from build123d import *


# Not quite as in the source:
# - a fillet or chamfer that OpenCascade refuses, or shapes differently, is made with other operations: its cross-section is extruded or revolved along the edge and cut away or added


with BuildPart() as f1:
    # F0 (on Front) → F1 (revolve)
    with BuildSketch(Plane.XZ):
        with BuildLine():
            Line((-38.1, 0), (0, 0))
            Line((0, 0), (0, 27.2913607001))
            ThreePointArc((0, 27.2913607001), (-6.35, 33.6413607001), (0, 39.9913607001))
            Line((0, 39.9913607001), (0, 77.1941723466))
            ThreePointArc((0, 77.1941723466), (-6.35, 83.5441723466), (0, 89.8941723466))
            Line((0, 89.8941723466), (0, 101.6))
            Line((0, 101.6), (-38.1, 101.6))
            Line((-38.1, 101.6), (-38.1, 0))
        make_face()
    revolve(axis=Axis((-38.1, 0, 50.8), (0, 0, 1)))

    # F2: chamfer of 5.08 on 4 edges, made by hand

    # F2_s1 → F2_t2 (revolve, cut)
    with BuildSketch(Plane.XZ):
        Polygon((0, 96.52), (-5.08, 101.6), (0, 101.6), align=None)
    revolve(axis=Axis((-38.1, 0, 101.6), (0, 0, 1)), mode=Mode.SUBTRACT)

    # F2_s3 → F2_t4 (revolve, cut)
    with BuildSketch(Plane.XZ):
        Polygon((-5.08, 0), (0, 5.08), (0, 0), align=None)
    revolve(axis=Axis((-38.1, 0, 0), (0, 0, 1)), mode=Mode.SUBTRACT)

    # F2_s5 → F2_t6 (revolve, cut)
    with BuildSketch(Plane.XZ):
        with BuildLine():
            Line((0, 23.4022933598), (-2.8222222222, 27.9529899555))
            ThreePointArc((-2.8222222222, 27.9529899555), (-1.5219513398, 27.4764467413), (0, 27.2913607001))
            Line((0, 27.2913607001), (0, 23.4022933598))
        make_face()
    revolve(axis=Axis((-38.1, 0, 27.2913607001), (0, 0, 1)), mode=Mode.SUBTRACT)


solid = f1.part
Can you work these out from the model? Positions are in its coordinate system, mm. Coordinates: 2 decimals unless noted, no trailing zeros. Loops run counter-clockwise (first coordinate to the right, second up) from the corner with the lowest first, then second, coordinate; pieces in that order, holes last. Notation, with made-up numbers: (46, 77) - (81, 77) arc R25 ccw to (81, 96) - close; hole circle Ø1 at (42, 36.5). An arc over 180 degrees is marked (long way). Answer as a JSON object with one key per item and string values. Group by question number.
Item 1: If we section it at B-B (x = -38.1): List the corners of the cut face in (y, z) for me.
Item 2: If we mould it in two halves opening along Z, with no side actions, what happens to faces 1 (the face through (-4.32, 10.64, 27.73)), 2 (the face through (-38, 0, 0)), 3 (the face through (-39, 0, 101.6)), 4 (the face through (-68.335, -23.183, 14.369))? For each: released by +Z, released by -Z, zero draft, split by the parting line, or undercut.
Item 3: If I drill on L1, parallel to Z at x = -18, y = 32; L2, parallel to Z at x = -71, y = -15; L3, parallel to X at y = -1.5, z = 69.5, over which ranges is the centre line in solid material (lowest first)? Write a range as from..to.
Item 4: If we section it at A-A (y = 0): List the corners of the cut face in (x, z) for me, plus the area to 3 significant figures.
Item 5: For pin 1 (1.5 mm diameter, centred on x = -42.5, z = 76, fed in from +Y); pin 2 (2 mm diameter, centred on x = -53, z = 30, fed in from +Y); pin 3 (6 mm diameter, centred on x = -59, z = 84.5, fed in from -Y), each with a flat end and sliding along its axis, tell me the tip position at first contact or that it passes through.
Item 6: If we section it at C-C (z = 73): List the corners of the cut face in (x, y) for me, plus the area to 3 significant figures.
Returned:
{
 "1": {"outline": "(-38.1, 5.08) - (-33.02, 0) - (33.02, 0) - (38.1, 5.08) - (38.1, 23.4) - (35.28, 27.95) arc R6.35 cw to (38.1, 39.99) - (38.1, 77.19) arc R6.35 cw to (38.1, 89.89) - (38.1, 96.52) - (33.02, 101.6) - (-33.02, 101.6) - (-38.1, 96.52) - (-38.1, 89.89) arc R6.35 cw to (-38.1, 77.19) - (-38.1, 39.99) arc R6.35 cw to (-35.28, 27.95) - (-38.1, 23.4) - close"},
 "2": {"face 1": "undercut", "face 2": "released by -Z", "face 3": "released by +Z", "face 4": "zero draft"},
 "3": {"L1": "z = 4.77..23.9, 39.98..77.2, 89.89..96.83", "L2": "z = 3.14..26.53, 39.69..77.5, 89.59..98.46", "L3": "x = -76.17..-0.03"},
 "4": {"outline": "(-76.2, 5.08) - (-71.12, 0) - (-5.08, 0) - (0, 5.08) - (0, 23.4) - (-2.82, 27.95) arc R6.35 cw to (0, 39.99) - (0, 77.19) arc R6.35 cw to (0, 89.89) - (0, 96.52) - (-5.08, 101.6) - (-71.12, 101.6) - (-76.2, 96.52) - (-76.2, 89.89) arc R6.35 cw to (-76.2, 77.19) - (-76.2, 39.99) arc R6.35 cw to (-73.38, 27.95) - (-76.2, 23.4) - close", "area": "7,430 mm²"},
 "5": {"pin 1": "stops at y = 37.92", "pin 2": "stops at y = 30.4", "pin 3": "stops at y = -26.58"},
 "6": {"outline": "circle Ø76.2 at (-38.1, 0)", "area": "4,560 mm²"}
}
